Here's the drawing with two shaded views (mm, measured from the low corner). I have some questions. Round coordinates to 2 decimals unless told otherwise and drop trailing zeros. Order: outer loops, then holes, each group sorted by start corner. A loop starts at its lowest first (then second) coordinate and runs counter-clockwise, first axis right, second up. Notation, with made-up numbers: (31.5, -10) - (81.5, -10) arc R8 ccw to (81.5, 1) - close; hole circle Ø1 at (14, -28). An arc over 180 degrees is marked (long way). Return JSON: item names as keys, results as strings. Group by question number.
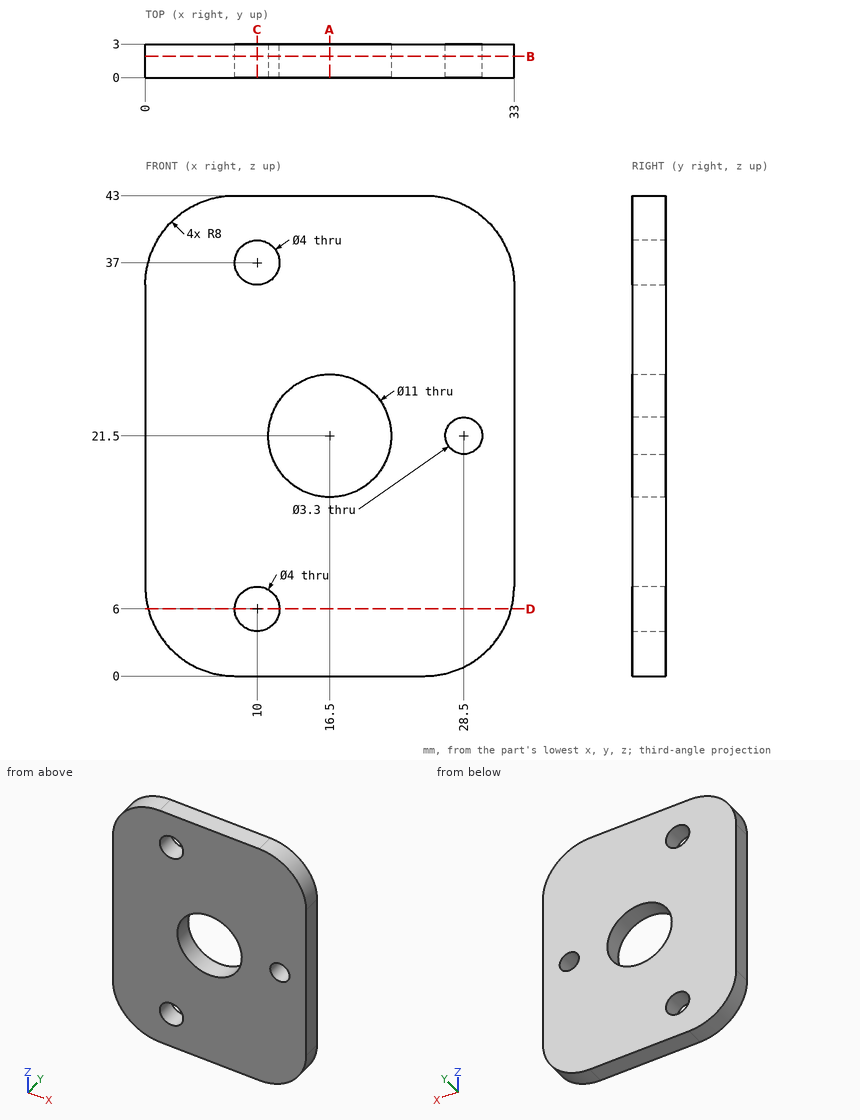
1) I want a section at A-A, the plane x = 16.5. List the corners of the cut face in (y, z) for me, plus the area to 3 significant figures.
2) I want a section at D-D, the plane z = 6. List the corners of the cut face in (x, y) for me.
3) I want a section at C-C, the plane x = 10. List the corners of the cut face in (y, z) for me.
4) If I drill on line 1 along X through (y, z) = (1.3, 21.5); line 2 along X through (y, z) = (0.3, 20); line 3 along X through (y, z) = (1.9, 6), over which ranges is the centre line in solid material (lowest first)? Write a range as from..to.
5) I want a section at B-B, the plane y = 1.9. List the corners of the cut face in (x, z) for me.
Outcome:
{
 "1": {"outline": "(0, 0) - (3, 0) - (3, 16) - (0, 16) - close; (0, 27) - (3, 27) - (3, 43) - (0, 43) - close", "area": "96.0 mm^2"},
 "2": {"outline": "(0.25, 0) - (8, 0) - (8, 3) - (0.25, 3) - close; (12, 0) - (32.75, 0) - (32.75, 3) - (12, 3) - close"},
 "3": {"outline": "(0, 0) - (3, 0) - (3, 4) - (0, 4) - close; (0, 8) - (3, 8) - (3, 35) - (0, 35) - close; (0, 39) - (3, 39) - (3, 43) - (0, 43) - close"},
 "4": {"line 1": "0..11, 22..26.85, 30.15..33", "line 2": "0..11.21, 21.79..27.81, 29.19..33", "line 3": "0.25..8, 12..32.75"},
 "5": {"outline": "(0, 8) arc R8 ccw to (8, 0) - (25, 0) arc R8 ccw to (33, 8) - (33, 35) arc R8 ccw to (25, 43) - (8, 43) arc R8 ccw to (0, 35) - close; hole circle Ø4 at (10, 6); hole circle Ø4 at (10, 37); hole circle Ø11 at (16.5, 21.5); hole circle Ø3.3 at (28.5, 21.5)"}
}
